Job drawing, mm, ordinate dimensions from the low corner. One solid piece. Round coordinates to 2 decimals unless told otherwise and drop trailing zeros. Loops run counter-clockwise (first coordinate to the right, second up) from the corner with the lowest first, then second, coordinate; pieces in that order, holes last.
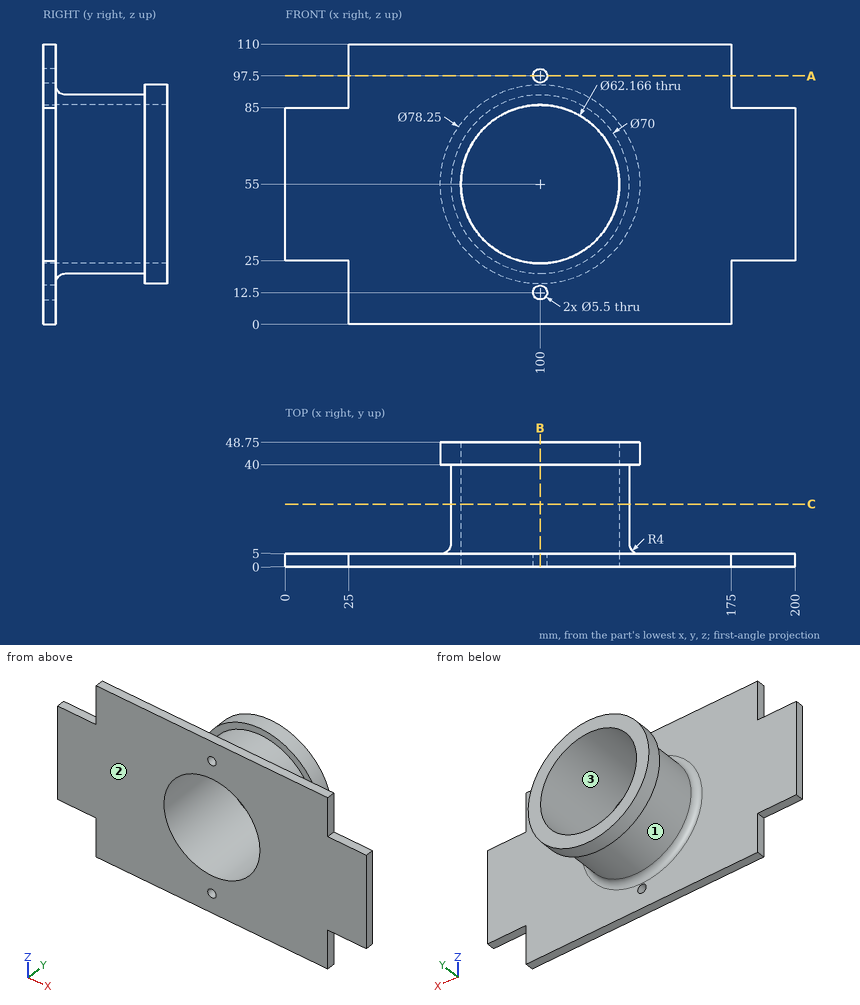
(1) Probe line 1 (X direction, y = 3.65, z = 12.5); line 2 (X direction, y = 19.5, z = 55); line 3 (Y direction, x = 67, z = 84.5). List the from-to ranges inside material, lowest first.
Responses:
line 1: x = 25 to 97.25, 102.75 to 175
line 2: x = 65 to 68.92, 131.08 to 135
line 3: y = 0 to 5
(2) Slice it at A-A on z = 97.5. List the corners of the cut face in (x, y).
Responses:
outline: (25, 0) - (97.25, 0) - (97.25, 5) - (25, 5) - close; (102.75, 0) - (175, 0) - (175, 5) - (102.75, 5) - close
(3) Pull direction Y, two halves, no side cores. Call the marked faces 1, 2 and 3: +Y half, -Y half, draft (parallel to the pull), parting line (faces both ways), or undercut.
Responses:
face 1: undercut
face 2: -Y half
face 3: draft
(4) Slice it at B-B on x = 100. Count the separate pieces of the cut face and the enclosed holes in it, plus the area to 3 significant figures.
Responses:
separate pieces: 4
enclosed holes: 0
area: 606 mm2
(5) Pin check, flat tips, straight feed: P1, Ø9, axis at x = 100, z = 97.5, coming from the -Y side; P2, Ø5.5, axis at x = 192, y = 2.5, coming from the -Z side; P3, Ø2.5, axis at y = 2, z = 11.5, coming from the -X side; P4, Ø6, axis at x = 102, z = 29, coming from the -Y side (1 decimal). Stop position of each tip, or through.
Responses:
P1: stops at y = 0
P2: stops at z = 25
P3: stops at x = 25
P4: passes through
(6) Slice it at C-C on y = 24.5. List the corners of the cut face in (x, z), plus the area to 3 significant figures.
Responses:
outline: circle Ø70 at (100, 55); hole circle Ø62.17 at (100, 55)
area: 813 mm2
